Build history of the part. All positions in model axes, mm. A direction names the side the tool comes from. Round coordinates to 2 decimals unless told otherwise and drop trailing zeros. Write each loop counter-clockwise with the first axis right and the second up, starting at its lowest first coordinate (ties: lowest second). Pieces come first, ordered by that corner, then holes. Notation, with made-up numbers: M 56,7.25 L 96,7.25 A6 cw 96,17.25 Z; hole C -38,28.25 d4. An arc over 180 degrees is marked long. Write item = value, one per line.
from build123d import *

# Parameters (mm, degrees)
BOSS_EXTRUDE1_DEPTH                       = 43.942
CUT_EXTRUDE1_START                        = -40.767
CUT_EXTRUDE1_DEPTH                        = 40.767
FILLET1_R                                 = 1.27
CSK_FOR_4_FLAT_HEAD_MACHINE_SCREW_2_COUNT = 2
CSK_FOR_4_FLAT_HEAD_MACHINE_SCREW_2_PITCH = 17.1196
CUT_EXTRUDE2_DEPTH                        = 75.354351507
FILLET3_R                                 = 1.778
FILLET4_R                                 = 1.27
FILLET5_R                                 = 6.35
SKETCH8_R                                 = 1.651
CUT_EXTRUDE3_DEPTH                        = 40.767


with BuildPart() as part:
    # Sketch1 → Boss-Extrude1 (new body)
    with BuildSketch(Plane(origin=(0, 0, 0), x_dir=(1, 0, 0), z_dir=(0, 1, 0))):
        with BuildLine():
            Line((12.192, 26.67), (12.192, 0.545071947))
            ThreePointArc((12.192, 0.545071947), (16.556076609, -5.486396223), (12.192, -11.517864393))
            Line((12.192, -11.517864393), (12.192, -26.67))
            Line((12.192, -26.67), (16.9545, -26.67))
            Line((16.9545, -26.67), (16.9545, -19.977285695))
            Line((16.9545, -19.977285695), (16.9545, -18.510549526))
            ThreePointArc((16.9545, -18.510549526), (27.432, 0), (16.9545, 18.510549526))
            Line((16.9545, 18.510549526), (16.9545, 19.977285695))
            Line((16.9545, 19.977285695), (16.9545, 26.67))
            Line((16.9545, 26.67), (12.192, 26.67))
        make_face()
    extrude(amount=-BOSS_EXTRUDE1_DEPTH)

    # Sketch3 → Cut-Extrude1 (cut)
    with BuildSketch(Plane.XZ.offset(43.942).offset(CUT_EXTRUDE1_START)):
        with BuildLine():
            ThreePointArc((12.192, -17.016104372), (23.368, 0), (12.192, 17.016104372))
            Line((12.192, 17.016104372), (12.192, 11.517864393))
            ThreePointArc((12.192, 11.517864393), (16.556076609, 5.486396223), (12.192, -0.545071947))
            Line((12.192, -0.545071947), (12.192, -17.016104372))
        make_face()
    extrude(amount=CUT_EXTRUDE1_DEPTH, mode=Mode.SUBTRACT)

    # Fillet1
    fillet1_edges = [part.edges().sort_by_distance(p)[0] for p in [
        (12.192, -1.5875, -0.545071947),
        (12.192, -1.5875, 11.517864393),
    ]]
    fillet(fillet1_edges, radius=FILLET1_R)

    # Sketch6 → CSK for #4 Flat Head Machine Screw (100)1 (revolve, cut)
    with BuildSketch(Plane(origin=(16.9545, -9.525, 22.606), x_dir=(0, 0, -1), z_dir=(0, 1, 0))):
        Polygon((0, 0), (0, 7.838574487), (1.63195, 6.858), (1.63195, 1.028358553), (2.8575, 0), align=None)
    csk_for_4_flat_head_machine_screw_100 = revolve(axis=Axis((23.3045, -9.525, 22.606), (-1, 0, 0)), mode=Mode.SUBTRACT)

    # CSK for _4 Flat Head Machine Screw _ 2: CSK for #4 Flat Head Machine Screw (100)1 ×2
    with Locations(*[(0, -i * CSK_FOR_4_FLAT_HEAD_MACHINE_SCREW_2_PITCH, 0) for i in range(1, CSK_FOR_4_FLAT_HEAD_MACHINE_SCREW_2_COUNT)]):
        add(csk_for_4_flat_head_machine_screw_100, mode=Mode.SUBTRACT)

    # Mirror1: CSK for #4 Flat Head Machine Screw (100)1 across plane
    add(csk_for_4_flat_head_machine_screw_100.mirror(Plane.XY), mode=Mode.SUBTRACT)

    # Mirror1 copy 1 sketch → Mirror1 copy 1 (revolve, cut)
    with BuildSketch(Plane(origin=(16.9545, -26.6446, -22.606), x_dir=(0, 0, 1), z_dir=(0, 1, 0))):
        Polygon((0, 0), (0, -7.838574487), (1.63195, -6.858), (1.63195, -1.028358553), (2.8575, 0), align=None)
    revolve(axis=Axis((23.3045, -26.6446, -22.606), (1, 0, 0)), mode=Mode.SUBTRACT)

    # Sketch7 → Cut-Extrude2 (cut, through all)
    with BuildSketch(Plane.XY.offset(26.67)):
        Polygon((12.192, -37.563057674), (29.718, -43.942), (12.192, -43.942), align=None)
    extrude(amount=-CUT_EXTRUDE2_DEPTH, mode=Mode.SUBTRACT)

    # Fillet3
    fillet3_edges = [part.edges().sort_by_distance(p)[0] for p in [
        (16.9545, -19.648232957, -18.510549526),
        (16.9545, -19.648232957, 18.510549526),
    ]]
    fillet(fillet3_edges, radius=FILLET3_R)

    # Fillet4
    # the kernel refuses this fillet: 1.27 mm, written as the material it takes off along each edge
    with BuildSketch(Plane(origin=(15.6845, -1.27, -25.4), x_dir=(0, 0, -1), z_dir=(1, 0, 0))) as fillet4_piece_1_section:
        Polygon((0, 0), (FILLET4_R, 0), (FILLET4_R, FILLET4_R), (0, FILLET4_R), align=None)
    fillet4_piece_1 = extrude(amount=FILLET4_R, mode=Mode.PRIVATE)
    fillet4_piece_1 = fillet4_piece_1 - Plane(origin=(15.6845, -1.27, -25.4), x_dir=(0, -0.7071067811865475, 0.7071067811865475), z_dir=(1, 0, 0)) * Sphere(FILLET4_R, mode=Mode.PRIVATE)
    add(fillet4_piece_1, mode=Mode.SUBTRACT)
    with BuildSketch(Plane(origin=(15.6845, -1.27, 25.4), x_dir=(1, 0, 0), z_dir=(0, 0, 1))) as fillet4_piece_2_section:
        Polygon((0, 0), (FILLET4_R, 0), (FILLET4_R, FILLET4_R), (0, FILLET4_R), align=None)
    fillet4_piece_2 = extrude(amount=FILLET4_R, mode=Mode.PRIVATE)
    fillet4_piece_2 = fillet4_piece_2 - Plane(origin=(15.6845, -1.27, 25.4), x_dir=(-0.7071067811865475, -0.7071067811865475, 0), z_dir=(0, 0, 1)) * Sphere(FILLET4_R, mode=Mode.PRIVATE)
    add(fillet4_piece_2, mode=Mode.SUBTRACT)
    with BuildSketch(Plane(origin=(15.6845, 0, -26.67), x_dir=(0, -1, 0), z_dir=(-1, 0, 0)), Plane(origin=(9.017, 0, 26.67), x_dir=(0, -1, 0), z_dir=(1, 0, 0))) as fillet4_piece_3:
        with BuildLine():
            CenterArc((FILLET4_R, FILLET4_R), FILLET4_R, 180, 90)
            Line((0, FILLET4_R), (0, 0))
            Line((0, 0), (FILLET4_R, 0))
        make_face()
    extrude(amount=6.6675, mode=Mode.SUBTRACT)
    with BuildSketch(Plane(origin=(5.842, 0, 0), x_dir=(0.5516304347826092, 0, 0.8340886424245023), z_dir=(-0.8340886424245023, 0, 0.5516304347826092))) as fillet4_piece_4:
        with BuildLine():
            CenterArc((21.59 - FILLET4_R, -FILLET4_R), FILLET4_R, 0, 90)
            Line((21.59 - FILLET4_R, 0), (21.59, 0))
            Line((21.59, 0), (21.59, -FILLET4_R))
        make_face()
    revolve(axis=Axis((5.842, 0, 0), (0, 1, 0)), revolution_arc=113.042120672, mode=Mode.SUBTRACT)
    with BuildSketch(Plane(origin=(16.9545, 0, -25.4), x_dir=(0, -1, 0), z_dir=(0, 0, 1)), Plane(origin=(16.9545, 0, 19.490983396), x_dir=(0, -1, 0), z_dir=(0, 0, 1))) as fillet4_piece_5:
        with BuildLine():
            CenterArc((FILLET4_R, -FILLET4_R), FILLET4_R, 90, 90)
            Line((0, -FILLET4_R), (0, 0))
            Line((0, 0), (FILLET4_R, 0))
        make_face()
    extrude(amount=5.909016604, mode=Mode.SUBTRACT)
    with BuildSketch(Plane(origin=(18.7325, 0, -19.490983396), x_dir=(-0.5516304347826076, 0, 0.8340886424245035), z_dir=(0.8340886424245035, 0, 0.5516304347826076))) as fillet4_piece_6:
        with BuildLine():
            CenterArc((1.778 + FILLET4_R, FILLET4_R), FILLET4_R, 180, 90)
            Line((1.778 + FILLET4_R, 0), (1.778, 0))
            Line((1.778, 0), (1.778, FILLET4_R))
        make_face()
    revolve(axis=Axis((18.7325, 0, -19.490983396), (0, -1, 0)), revolution_arc=56.521060336, mode=Mode.SUBTRACT)
    with BuildSketch(Plane(origin=(18.7325, 0, 19.490983396), x_dir=(-1, 0, 0), z_dir=(0, 0, 1))) as fillet4_piece_7:
        with BuildLine():
            CenterArc((1.778 + FILLET4_R, FILLET4_R), FILLET4_R, 180, 90)
            Line((1.778 + FILLET4_R, 0), (1.778, 0))
            Line((1.778, 0), (1.778, FILLET4_R))
        make_face()
    revolve(axis=Axis((18.7325, 0, 19.490983396), (0, -1, 0)), revolution_arc=56.521060336, mode=Mode.SUBTRACT)
    with BuildSketch(Plane(origin=(16.9545, -1.27, 26.67), x_dir=(0, 0, -1), z_dir=(0, -1, 0))) as fillet4_piece_8:
        with BuildLine():
            CenterArc((FILLET4_R, -FILLET4_R), FILLET4_R, 90, 90)
            Line((0, -FILLET4_R), (0, 0))
            Line((0, 0), (FILLET4_R, 0))
        make_face()
    extrude(amount=41.201465915, mode=Mode.SUBTRACT)
    with BuildSketch(Plane(origin=(16.9545, -1.27, -26.67), x_dir=(0, 0, 1), z_dir=(0, -1, 0))) as fillet4_piece_9:
        with BuildLine():
            CenterArc((FILLET4_R, FILLET4_R), FILLET4_R, 180, 90)
            Line((0, FILLET4_R), (0, 0))
            Line((0, 0), (FILLET4_R, 0))
        make_face()
    extrude(amount=41.201465915, mode=Mode.SUBTRACT)

    # Fillet5
    fillet5_edges = [part.edges().sort_by_distance(p)[0] for p in [
        (12.192, -37.563057674, -21.843052186),
        (12.192, -37.563057674, 21.843052186),
    ]]
    fillet(fillet5_edges, radius=FILLET5_R)

    # Sketch8 → Cut-Extrude3 (cut)
    with BuildSketch(Plane(origin=(0, 0, 0), x_dir=(1, 0, 0), z_dir=(0, 1, 0))):
        with Locations(Location((17.967730782, 9.64524178, 0), (0, 0, 270))):
            Circle(SKETCH8_R)
        with Locations(Location((20.257889798, -5.678570007, 0), (0, 0, 270))):
            Circle(SKETCH8_R)
    extrude(amount=-CUT_EXTRUDE3_DEPTH, mode=Mode.SUBTRACT)


solid = part.part
1. Flat gauge pins, fed straight in: pin 1 (4.5 mm diameter, centred on y = -17, z = 23, fed in from +X); pin 2 (2 mm diameter, centred on y = -26.64, z = 22.61, fed in from +X); pin 3 (8 mm diameter, centred on x = 24, y = -6, fed in from -Z); pin 4 (5.5 mm diameter, centred on x = 19.5, z = 1, fed in from -Y) (3 decimals). Where does each tip first touch, or does it go through?
Responses:
pin_1 = 16.95
pin_2 = through
pin_3 = -16.3
pin_4 = -3.175
2. Band-saw the part on B-B (y = -14). List the corners of the cut face in (x, z).
Responses:
outline = M 12.19,-26.67 L 15.68,-26.67 A1.27 ccw 16.95,-25.4 L 16.95,-19.49 A1.78 cw 17.75,-18.01 A21.59 ccw 17.75,18.01 A1.78 cw 16.95,19.49 L 16.95,25.4 A1.27 ccw 15.68,26.67 L 12.19,26.67 L 12.19,17.02 A18.54 cw 12.19,-17.02 Z
3. Mould opens along Z. For faces 4 (the face through (16.59, -0.38, 22.4)), 5 (the face through (14, -20, 26.67)), 6 (the face through (14.09, -25.05, -22.96)) say: pulls with the +Z half, pulls with the -Z half, needs draft (parallel to the pull), parting line crosses it, or undercut.
Responses:
face_4 = needs draft
face_5 = pulls with the +Z half
face_6 = undercut
4. Probe probe 1 along Y at (x, z) = (13, 21.5); probe 2 along Z at (x, y) = (19, -35); probe 3 along Y at (x, z) = (16.25, 9) (3 decimals). List the from-to ranges inside material, lowest first.
Responses:
probe_1 = -36.22 to -27.84, -25.44 to -10.73, -8.32 to 0
probe_2 = -17.12 to -11.95, 11.95 to 17.12
probe_3 = -3.175 to 0
5. Tool access for faces 1 (the face through (23.366, -22.334, -0.302)), 2 (the face through (16.954, -20, -22)), 3 (the face through (12.384, -1.61, -0.732)): list every direction of +Z, -Z, +X, -X, +Y, -Y with a clear straight run to the whole face (end or side of a thin tool).
Responses:
face_1 = -X, -Y
face_2 = -Z, +X, +Y, -Y
face_3 = -X, +Y, -Y
6. Band-saw the part on C-C (y = -37.5). List the corners of the cut face in (x, z), plus the area to 3 significant figures.
Responses:
outline = M 13.95,-26.67 L 15.68,-26.67 A1.27 ccw 16.95,-25.4 L 16.95,-19.49 A1.78 cw 17.75,-18.01 A21.59 ccw 17.75,18.01 A1.78 cw 16.95,19.49 L 16.95,25.4 A1.27 ccw 15.68,26.67 L 13.95,26.67 L 13.95,16.14 A18.54 cw 13.95,-16.14 Z
area = 218 mm²
7. Band-saw the part on A-A (x = 13.75). List the corners of the cut face in (y, z) (3 decimals).
Responses:
outline = M -37.283,-26.67 L -1.27,-26.67 A1.27 ccw 0,-25.4 L 0,0.217 L -3.175,0.217 L -3.175,-16.253 L -37.283,-16.253 Z; M -37.283,16.253 L -3.175,16.253 L -3.175,10.755 L 0,10.755 L 0,25.4 A1.27 ccw -1.27,26.67 L -37.283,26.67 Z; hole C -26.645,-22.606 d3.264; hole C -26.645,22.606 d3.264; hole C -9.525,-22.606 d3.264; hole C -9.525,22.606 d3.264
